```python
from build123d import *

# Parameters (mm, degrees)
F1_W     = 15
F1_H     = 15
F1_W_2   = 13
F1_H_2   = 13
F2_DEPTH = 250
F4_DEPTH = 25


with BuildPart() as f2:
    # F1 (on Top) → F2 (new body)
    with BuildSketch(Plane.XY):
        Rectangle(F1_W, F1_H)
        Rectangle(F1_W_2, F1_H_2, mode=Mode.SUBTRACT)
    extrude(amount=F2_DEPTH)

    # F3 (on face) → F4 (cut)
    with BuildSketch(Plane.XZ.offset(7.5)):
        Polygon((7.5, 6.2132034356), (-7.5, 0), (7.5, 0), align=None)
        Polygon((7.5, 250), (-7.5, 250), (7.5, 243.7867965644), align=None)
    extrude(amount=-F4_DEPTH, mode=Mode.SUBTRACT)


solid = f2.part
```
Here's how the part is built. I have some questions about the finished solid (model axes, mm). A direction names the side the tool comes from. Give positions to 0.01 mm unless a question says otherwise; leave off trailing zeros. Order: outer loops, then holes, each group sorted by start corner. A loop starts at its lowest first (then second) coordinate and runs counter-clockwise, first axis right, second up. Notation, with made-up numbers: M -33,21 L -18,21 A37 cw -18,59 Z; hole C 17.25,-33.5 d10. An arc over 180 degrees is marked long. Use a Markdown table: item, result. Add a question column.
1. Suppose I cut it at C-C (x = 4). List the corners of the cut face in (y, z) for me.
2. On a 3-axis mill with a long thin cutter (end or side, diameter ignored), from which of +Z, -Z, +X, -X, +Y, -Y can I reach the whole of each face in a straight line? I mean faces 1 (the flat face through (-7.5, 0, 123)), 2 (the flat face through (0, -6.5, 123)). Say none if no direction works.
3. If we mould it in two halves opening along Y, with no side actions, what happens to faces 3 (the flat face through (0, -7.5, 123)), 4 (the flat face through (-0.105, -6.772, 246.937)), 5 (the flat face through (-6.5, 0, 123)), 6 (the flat face through (0, 7.5, 123))? For each: +Y half, -Y half, draft (parallel to the pull), parting line (faces both ways), or undercut.
4. For pin 1 Ø6 at (x, y) = (5, -1) entering from -Z, with a flat end and sliding along its axis, tell me the tip position at first contact or that it passes through.
5. Suppose I cut it at A-A (y = -3.75). List the corners of the cut face in (x, z) for me, and give its area (3 significant figures).
6. I need wall thicknesses on probe 1 along Y at (x, z) = (0, 42.5); probe 2 along Z at (x, y) = (-4.5, 6.75). Which ranges of each line are inside material? Lowest first, please. Write a range as from..to.
7. Suppose I cut it at B-B (z = 42). List the corners of the cut face in (x, y) for me.
Results list:
| question | item | result |
|---|---|---|
| 1 | outline | M -7.5,4.76 L -6.5,4.76 L -6.5,245.24 L -7.5,245.24 Z; M 6.5,4.76 L 7.5,4.76 L 7.5,245.24 L 6.5,245.24 Z |
| 2 | face 1 | +Z, -Z, -X, +Y, -Y |
| 2 | face 2 | +Z, -Z |
| 3 | face 3 | -Y half |
| 3 | face 4 | draft |
| 3 | face 5 | undercut |
| 3 | face 6 | +Y half |
| 4 | pin 1 | stops at z = 5.8 |
| 5 | outline | M -7.5,0 L -6.5,0.41 L -6.5,249.59 L -7.5,250 Z; M 6.5,5.8 L 7.5,6.21 L 7.5,243.79 L 6.5,244.2 Z |
| 5 | area | 488 mm² |
| 6 | probe 1 | y = -7.5..-6.5, 6.5..7.5 |
| 6 | probe 2 | z = 1.24..248.76 |
| 7 | outline | M -7.5,-7.5 L 7.5,-7.5 L 7.5,7.5 L -7.5,7.5 Z; hole M -6.5,-6.5 L 6.5,-6.5 L 6.5,6.5 L -6.5,6.5 Z |
